from build123d import *

# Parameters (mm, degrees)
F1_DEPTH    = 22.225
F2_R        = 7.62
F3_T1_DEPTH = 47.5792387778
F4_R        = 3.2639
F5_DEPTH    = 4.7762
F6_R        = 4.1656
F7_DEPTH    = 4.7762


# Not quite as in the source:
# - a fillet or chamfer that OpenCascade refuses, or shapes differently, is made with other operations: its cross-section is extruded or revolved along the edge and cut away or added


with BuildPart() as f1:
    # F0 (on Right) → F1 (new body)
    with BuildSketch(Plane.YZ):
        Polygon((0, 38.1), (0, 0), (38.1, 0), (38.1, 4.7752), (4.7752, 4.7752), (4.7752, 38.1), align=None)
    extrude(amount=-F1_DEPTH)

    # F2
    f2_edges = [f1.edges().sort_by_distance(p)[0] for p in [
        (-11.1125, 4.7752, 4.7752),
    ]]
    fillet(f2_edges, radius=F2_R)

    # F3: fillet of radius 5.08 on 2 edges, made by hand

    # F3_s2 → F3_t1 (cut)
    with BuildSketch(Plane.YZ.offset(-34.9021193889)):
        with BuildLine():
            ThreePointArc((4.7752, 33.0291522444), (3.3934958238, 36.5118247815), (0, 38.1))
            Line((0, 38.1), (4.7752, 38.1))
            Line((4.7752, 38.1), (4.7752, 33.0291522444))
        make_face()
        with BuildLine():
            ThreePointArc((33.0291522444, 4.7752), (36.5118247815, 3.3934958238), (38.1, 0))
            Line((38.1, 0), (38.1, 4.7752))
            Line((38.1, 4.7752), (33.0291522444, 4.7752))
        make_face()
    extrude(amount=F3_T1_DEPTH, mode=Mode.SUBTRACT)

    # F4 (on face) → F5 (cut, through all)
    with BuildSketch(Plane(origin=(0, 4.7752, 0), x_dir=(-1, 0, 0), z_dir=(0, 1, 0))):
        with Locations((11.1125, 19.05)):
            Circle(F4_R)
    extrude(amount=-F5_DEPTH, mode=Mode.SUBTRACT)

    # F6 (on face) → F7 (cut, through all)
    with BuildSketch(Plane.XY.offset(4.7752)):
        with Locations((-11.1125, 19.05)):
            Circle(F6_R)
    extrude(amount=-F7_DEPTH, mode=Mode.SUBTRACT)


solid = f1.part
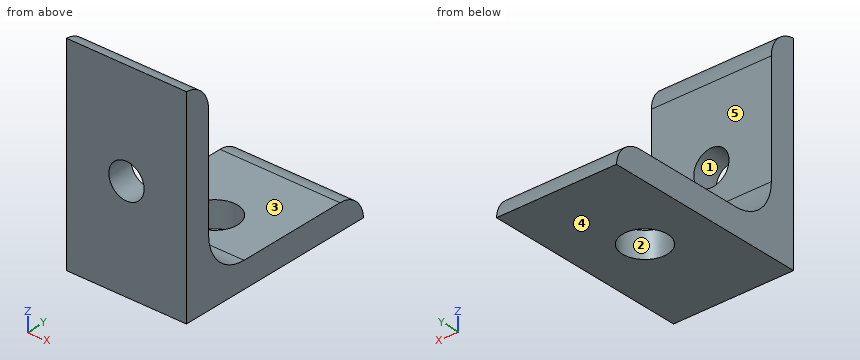
Can you work these out from the model? Positions are in its coordinate system, mm. Face numbers are marked on the shaded views. A direction names the side the tool comes from. Coordinates: 2 decimals unless noted, no trailing zeros. Order: outer loops, then holes, each group sorted by start corner. A loop starts at its lowest first (then second) coordinate and runs counter-clockwise, first axis right, second up. Notation, with made-up numbers: M 71,-36.5 L 130,-36.5 A13 ccw 130,-12.5 Z; hole C -4.5,-25 d1. An arc over 180 degrees is marked long. Write item = value, one per line.
(1) Suppose I cut it at D-D on x = -10.5. Please give me the cut outline in (y, z).
Results are:
outline = M 0,0 L 14.93,0 L 14.93,4.78 L 12.4,4.78 A7.62 cw 4.78,12.4 L 4.78,15.84 L 0,15.84 Z; M 0,22.26 L 4.78,22.26 L 4.78,33.03 A5.08 ccw 0,38.1 Z; M 23.17,0 L 38.1,0 A5.08 ccw 33.03,4.78 L 23.17,4.78 Z
(2) Suppose I cut it at B-B on y = 19.05. Please give me the cut outline in (x, z) (3 decimals), plus the area to 3 significant figures.
Results are:
outline = M -22.225,0 L -15.278,0 L -15.278,4.775 L -22.225,4.775 Z; M -6.947,0 L 0,0 L 0,4.775 L -6.947,4.775 Z
area = 66.3 mm2
(3) Suppose I cut it at C-C on x = -19.25. Please give me the cut outline in (y, z), plus the area to 3 significant figures.
Results are:
outline = M 0,0 L 38.1,0 A5.08 ccw 33.03,4.78 L 12.4,4.78 A7.62 cw 4.78,12.4 L 4.78,33.03 A5.08 ccw 0,38.1 Z
area = 343 mm2
(4) For the marked faces 4 and 5, which set-ups out of +Z, -Z, +X, -X, +Y, -Y let a thin tool reach every point of the face, with its end or its side?
Results are:
face_4 = -Z, +X, -X, +Y, -Y
face_5 = +Z, +X, -X, +Y
(5) Suppose I cut it at A-A on z = 19.05. Please give me the cut outline in (x, y) (3 decimals), plus the area to 3 significant figures.
Results are:
outline = M -22.225,0 L -14.376,0 L -14.376,4.775 L -22.225,4.775 Z; M -7.849,0 L 0,0 L 0,4.775 L -7.849,4.775 Z
area = 75.0 mm2
(6) If we mould it in two halves opening along Z, with no side actions, what happens to the marked faces 1, 2 and 3? For each: pulls with the +Z half, pulls with the -Z half, needs draft (parallel to the pull), parting line crosses it, or undercut.
Results are:
face_1 = undercut
face_2 = needs draft
face_3 = pulls with the +Z half
(7) For pin 1 Ø6 at (x, y) = (-12, 25) entering from +Z; pin 2 Ø5 at (x, z) = (-4.5, 14) entering from +Y, each with a flat end and sliding along its axis, tell me the tip position at first contact or that it passes through.
Results are:
pin_1 = 4.78
pin_2 = 4.83
(8) I need wall thicknesses on line 1 along X through (y, z) = (19, 3) (3 decimals); line 2 along Z through (x, y) = (-1, 19.5). Which ranges of each line are inside material? Lowest first, please. Write a range as [from, to].
Results are:
line_1 = [-22.225, -15.278], [-6.947, 0]
line_2 = [0, 4.78]
